Here's how the part is built. I have some questions about the finished solid (model axes, mm). Coordinates: 2 decimals unless noted, no trailing zeros. Order: outer loops, then holes, each group sorted by start corner. A loop starts at its lowest first (then second) coordinate and runs counter-clockwise, first axis right, second up. Notation, with made-up numbers: (-36.75, 41) -> (-28.75, 41) arc R21 cw to (-28.75, 66) -> close; hole circle Ø6 at (2.5, 30.25). An arc over 180 degrees is marked (long way). One line per item, written item: value. Start each with the question number.
```python
from build123d import *

# Parameters (mm, degrees)
SKETCH1_W                    = 59
SKETCH1_H                    = 87
BOSS_EXTRUDE1_DEPTH          = 1.5
CSK_FOR_M3_SFHCS1_AT_2_COUNT = 2
CSK_FOR_M3_SFHCS1_AT_2_PITCH = 78
CSK_FOR_M3_SFHCS1_AT_3_COUNT = 2
CSK_FOR_M3_SFHCS1_AT_3_PITCH = 92.649878575
CSK_FOR_M3_SFHCS1_AT_4_COUNT = 2
CSK_FOR_M3_SFHCS1_AT_4_PITCH = 50
FILLET3_R                    = 3
FILLET4_R                    = 0.5


with BuildPart() as part:
    # Sketch1 → Boss-Extrude1 (new, symmetric)
    with BuildSketch(Plane(origin=(0, 0, 0), x_dir=(1, 0, 0), z_dir=(0, 1, 0))):
        Rectangle(SKETCH1_W, SKETCH1_H)
    extrude(amount=BOSS_EXTRUDE1_DEPTH, both=True)

    # Sketch4 → CSK for M3 SFHCS1 (revolve, cut)
    with BuildSketch(Plane(origin=(-25, 1.5, -39), x_dir=(0, 0, 1), z_dir=(1, 0, 0))):
        Polygon((0, 0), (0, 3), (1.7, 3), (1.7, 1.66), (3.36, 0), align=None)
    csk_for_m3_sfhcs1 = revolve(axis=Axis((-25, 7.85, -39), (0, -1, 0)), mode=Mode.SUBTRACT)

    # CSK for M3 SFHCS1 at 2: CSK for M3 SFHCS1 ×2
    with Locations(*[(0, 0, i * CSK_FOR_M3_SFHCS1_AT_2_PITCH) for i in range(1, CSK_FOR_M3_SFHCS1_AT_2_COUNT)]):
        add(csk_for_m3_sfhcs1, mode=Mode.SUBTRACT)

    # CSK for M3 SFHCS1 at 3: CSK for M3 SFHCS1 ×2
    with Locations(*[Vector(0.5396661147204319, 0, 0.8418791389638739) * (i * CSK_FOR_M3_SFHCS1_AT_3_PITCH) for i in range(1, CSK_FOR_M3_SFHCS1_AT_3_COUNT)]):
        add(csk_for_m3_sfhcs1, mode=Mode.SUBTRACT)

    # CSK for M3 SFHCS1 at 4: CSK for M3 SFHCS1 ×2
    with Locations(*[(i * CSK_FOR_M3_SFHCS1_AT_4_PITCH, 0, 0) for i in range(1, CSK_FOR_M3_SFHCS1_AT_4_COUNT)]):
        add(csk_for_m3_sfhcs1, mode=Mode.SUBTRACT)

    # Fillet3
    fillet3_edges = [part.edges().sort_by_distance(p)[0] for p in [
        (29.5, 0, 43.5),
        (29.5, 0, -43.5),
    ]]
    fillet(fillet3_edges, radius=FILLET3_R)

    # Fillet4
    fillet4_edges = [part.edges().sort_by_distance(p)[0] for p in [
        (-1.5, 1.5, 43.5),
        (-1.5, 1.5, -43.5),
        (29.5, 1.5, 0),
        (28.621320344, 1.5, 42.621320344),
        (28.621320344, 1.5, -42.621320344),
    ]]
    fillet(fillet4_edges, radius=FILLET4_R)


solid = part.part
```
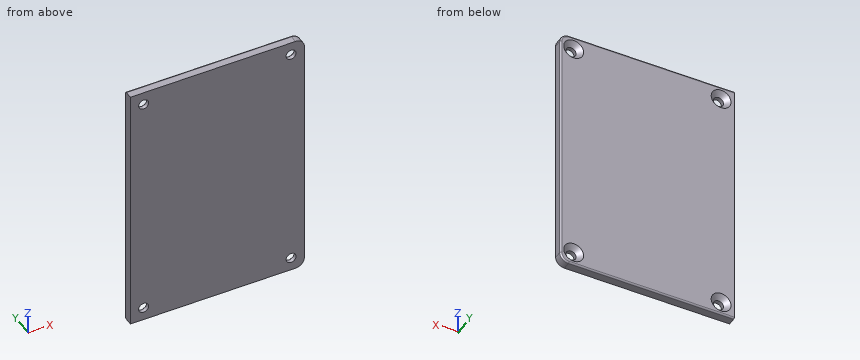
Q1. Imagine slicing it at A-A (x = -25). Write out the boundary of the cut face in (y, z).
Q2. Imagine slicing it at B-B (z = 39). Write out the boundary of the cut face in (x, y).
Q3. I need wall thicknesses on line 1 (X direction, y = -0.8, z = -39); line 2 (Z direction, x = -25, y = -0.5); line 3 (Z direction, x = 23, y = 0.9). Which ranges of each line are inside material? Lowest first, please.
Q4. For P1, Ø2.5, axis at x = -25, z = 39, coming from the -Y side; P2, Ø5.5, axis at x = 25, z = 39, coming from the +Y side; P3, Ø4.5, axis at x = 25, z = -39, coming from the -Y side, each with a flat end and sliding along its axis, tell me the tip position at first contact or that it passes through.
Completed:
1. outline: (-1.5, -43.5) -> (1, -43.5) arc R0.5 ccw to (1.5, -43) -> (1.5, -42.36) -> (-0.16, -40.7) -> (-1.5, -40.7) -> close; (-1.5, -37.3) -> (-0.16, -37.3) -> (1.5, -35.64) -> (1.5, 35.64) -> (-0.16, 37.3) -> (-1.5, 37.3) -> close; (-1.5, 40.7) -> (-0.16, 40.7) -> (1.5, 42.36) -> (1.5, 43) arc R0.5 ccw to (1, 43.5) -> (-1.5, 43.5) -> close
2. outline: (-29.5, -1.5) -> (-26.7, -1.5) -> (-26.7, -0.16) -> (-28.36, 1.5) -> (-29.5, 1.5) -> close; (-23.3, -1.5) -> (23.3, -1.5) -> (23.3, -0.16) -> (21.64, 1.5) -> (-21.64, 1.5) -> (-23.3, -0.16) -> close; (26.7, -1.5) -> (29.5, -1.5) -> (29.5, 1) arc R0.5 ccw to (29, 1.5) -> (28.36, 1.5) -> (26.7, -0.16) -> close
3. line 1: x = -29.5 to -26.7, -23.3 to 23.3, 26.7 to 29.5
3. line 2: z = -43.5 to -40.7, -37.3 to 37.3, 40.7 to 43.5
3. line 3: z = -43.5 to -40.9, -37.1 to 37.1, 40.9 to 43.5
4. P1: passes through
4. P2: stops at y = 0.89
4. P3: stops at y = -1.5
